Here's how the part is built. I have some questions about the finished solid (model axes, mm). Face numbers are marked on the shaded views. A direction names the side the tool comes from. Round coordinates to 2 decimals unless told otherwise and drop trailing zeros. Write each loop counter-clockwise with the first axis right and the second up, starting at its lowest first coordinate (ties: lowest second). Pieces come first, ordered by that corner, then holes. Notation, with made-up numbers: (30, 44.5) -> (52, 44.5) arc R19 cw to (52, 62.5) -> close; hole circle Ø2 at (81, 88.5). An arc over 180 degrees is marked (long way). Answer in a Markdown table with one row per item.
from build123d import *

# Parameters (mm, degrees)
SKETCH1_W            = 40
SKETCH1_H            = 30
BOSS_EXTRUDE1_DEPTH  = 5.5
SKETCH2_R            = 4.205
CUT_EXTRUDE1_DEPTH   = 44.072613109
M4_CLEARANCE_HOLE1_D = 4.5
SKETCH7_W            = 1.05
SKETCH7_H            = 20
CUT_EXTRUDE2_DEPTH   = 10


with BuildPart() as part:
    # Sketch1 → Boss-Extrude1 (new body)
    with BuildSketch(Plane.XY):
        Rectangle(SKETCH1_W, SKETCH1_H)
    extrude(amount=BOSS_EXTRUDE1_DEPTH)

    # Sketch2 → Cut-Extrude1 (cut, through all)
    with BuildSketch(Plane(origin=(20, 0, 0), x_dir=(0, 0, -1), z_dir=(1, 0, 0))):
        with Locations((0.3, 0)):
            Circle(SKETCH2_R)
    extrude(amount=-CUT_EXTRUDE1_DEPTH, mode=Mode.SUBTRACT)

    # M4 Clearance Hole1 (through all)
    with Locations(Plane.XY.offset(5.5)):
        with Locations((0, 10), (0, -10)):
            Hole(M4_CLEARANCE_HOLE1_D / 2)

    # Sketch7 → Cut-Extrude2 (cut)
    with BuildSketch(Plane(origin=(20, 0, 0), x_dir=(0, 0, -1), z_dir=(1, 0, 0))):
        with Locations((0.3, 0)):
            Rectangle(SKETCH7_W, SKETCH7_H)
    extrude(amount=-CUT_EXTRUDE2_DEPTH, mode=Mode.SUBTRACT)


solid = part.part
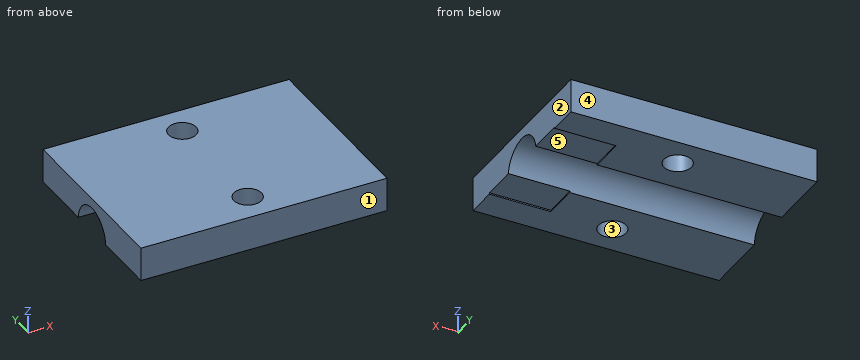
1) I need wall thicknesses on line 1 (Y direction, x = 0, z = 1.3); line 2 (Y direction, x = 1.5, z = 2.1); line 3 (Y direction, x = -17.5, z = 1.65). Which ranges of each line are inside material? Lowest first, please. Write a range as [from, to].
Response:
| item | result |
|---|---|
| line 1 | y = [-15, -12.25], [-7.75, -3.89], [3.89, 7.75], [12.25, 15] |
| line 2 | y = [-15, -11.68], [-8.32, -3.45], [3.45, 8.32], [11.68, 15] |
| line 3 | y = [-15, -3.73], [3.73, 15] |
2) For pin 1 (6.5 mm diameter, centred on x = 15, y = 6.5, fed in from -Z) (3 decimals), with a flat end and sliding along its axis, tell me the tip position at first contact or that it passes through.
Response:
| item | result |
|---|---|
| pin 1 | stops at z = 0.225 |
3) I want a section at A-A, the plane z = 3.15. List the corners of the cut face in (x, y) for me.
Response:
| item | result |
|---|---|
| outline | (-20, -15) -> (20, -15) -> (20, -2.4) -> (-20, -2.4) -> close; (-20, 2.4) -> (20, 2.4) -> (20, 15) -> (-20, 15) -> close; hole circle Ø4.5 at (0, -10); hole circle Ø4.5 at (0, 10) |
4) I want a section at C-C, the plane y = -11.75. List the corners of the cut face in (x, z) for me.
Response:
| item | result |
|---|---|
| outline | (-20, 0) -> (-1.41, 0) -> (-1.41, 5.5) -> (-20, 5.5) -> close; (1.41, 0) -> (20, 0) -> (20, 5.5) -> (1.41, 5.5) -> close |
5) We'd pull the mould along Y, two halves only. Please class the marked faces 1, 2 and 3: +Y half, -Y half, draft (parallel to the pull), parting line (faces both ways), or undercut.
Response:
| item | result |
|---|---|
| face 1 | -Y half |
| face 2 | draft |
| face 3 | undercut |
6) Which directions (+Z, -Z, +X, -X, +Y, -Y) give clear straight access to the entire face, cutting with the end or side of a thin tool? Please do the marked faces 4 and 5.
Response:
| item | result |
|---|---|
| face 4 | +Z, -Z, +X, -X, +Y |
| face 5 | -Z, +X |
7) I want a section at B-B, the plane x = 0. List the corners of the cut face in (y, z) for me (3 decimals).
Response:
| item | result |
|---|---|
| outline | (-15, 0) -> (-12.25, 0) -> (-12.25, 5.5) -> (-15, 5.5) -> close; (-7.75, 0) -> (-4.194, 0) arc R4.205 cw to (4.194, 0) -> (7.75, 0) -> (7.75, 5.5) -> (-7.75, 5.5) -> close; (12.25, 0) -> (15, 0) -> (15, 5.5) -> (12.25, 5.5) -> close |
8) I want a section at D-D, the plane x = 17. List the corners of the cut face in (y, z) for me (3 decimals), and give its area (3 significant figures).
Response:
| item | result |
|---|---|
| outline | (-15, 0) -> (-10, 0) -> (-10, 0.225) -> (-4.172, 0.225) arc R4.205 cw to (4.172, 0.225) -> (10, 0.225) -> (10, 0) -> (15, 0) -> (15, 5.5) -> (-15, 5.5) -> close |
| area | 137 mm^2 |
